CAD build for the part. Positions are in the model's coordinates, mm. Face numbers are marked on the shaded views. Coordinates: 2 decimals unless noted, no trailing zeros. Write each loop counter-clockwise with the first axis right and the second up, starting at its lowest first coordinate (ties: lowest second). Pieces come first, ordered by that corner, then holes.
```python
from build123d import *

# Parameters (mm, degrees)
SKETCH1_R           = 25
SKETCH1_R_2         = 15
BOSS_EXTRUDE1_DEPTH = 30
SKETCH2_R           = 30
BOSS_EXTRUDE2_DEPTH = 30
CUT_EXTRUDE1_START  = -30
SKETCH3_R           = 15
CUT_EXTRUDE1_DEPTH  = 30


with BuildPart() as part:
    # Sketch1 → Boss-Extrude1 (new body)
    with BuildSketch(Plane.XY):
        Circle(SKETCH1_R)
        Circle(SKETCH1_R_2, mode=Mode.SUBTRACT)
    extrude(amount=BOSS_EXTRUDE1_DEPTH)

    # Sketch2 → Boss-Extrude2 (add)
    with BuildSketch(Plane(origin=(0, 0, 0), x_dir=(-1, 0, 0), z_dir=(0, 0, -1))):
        Circle(SKETCH2_R)
    extrude(amount=BOSS_EXTRUDE2_DEPTH)

    # Sketch3 → Cut-Extrude1 (cut)
    with BuildSketch(Plane.XY.offset(CUT_EXTRUDE1_START)):
        Circle(SKETCH3_R)
    extrude(amount=CUT_EXTRUDE1_DEPTH, mode=Mode.SUBTRACT)


solid = part.part
```
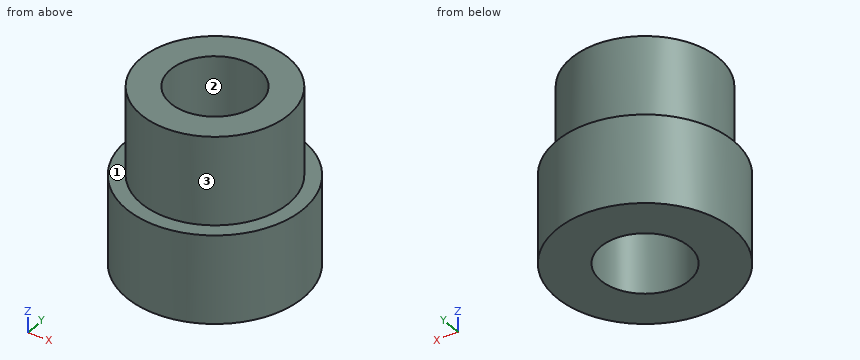
Item 1: Flat gauge pins, fed straight in: pin 1 Ø10 at (y, z) = (2.5, 22.5) entering from +X; pin 2 Ø6 at (x, z) = (11.5, 12.5) entering from +Y; pin 3 Ø1.5 at (x, z) = (15.5, -21.5) entering from -Y. Where does each tip first touch, or does it go through?
Item 2: Two-plate mould, pull along X, no slides. Class the marked faces 1, 2 and 3: +X half, -X half, draft (parallel to the pull), parting line (faces both ways), or undercut.
Item 3: Saw through at C-C, the plane z = -7.5. Write the cut outline in (x, y).
Item 4: Saw through at D-D, the plane y = 16.5. Write the cut outline in (x, z), and give its area (3 significant figures).
Item 5: Wall check: line 1 along Y through (x, z) = (0, -1); line 2 along Y through (x, z) = (0, 5); line 3 along Z through (x, y) = (25, -2.5). Give the ranges that are in metal, low to high.
Item 6: Saw through at A-A, the plane x = 0. Write the cut outline in (y, z).
Working result:
1. pin 1: stops at x = 25
1. pin 2: stops at y = 23.51
1. pin 3: stops at y = -26.12
2. face 1: draft
2. face 2: undercut
2. face 3: parting line
3. outline: circle Ø60 at (0, 0); hole circle Ø30 at (0, 0)
4. outline: (-25.05, -30) - (25.05, -30) - (25.05, 0) - (18.78, 0) - (18.78, 30) - (-18.78, 30) - (-18.78, 0) - (-25.05, 0) - close
4. area: 2,630 mm2
5. line 1: y = -30 to -15, 15 to 30
5. line 2: y = -25 to -15, 15 to 25
5. line 3: z = -30 to 0
6. outline: (-30, -30) - (-15, -30) - (-15, 30) - (-25, 30) - (-25, 0) - (-30, 0) - close; (15, -30) - (30, -30) - (30, 0) - (25, 0) - (25, 30) - (15, 30) - close
